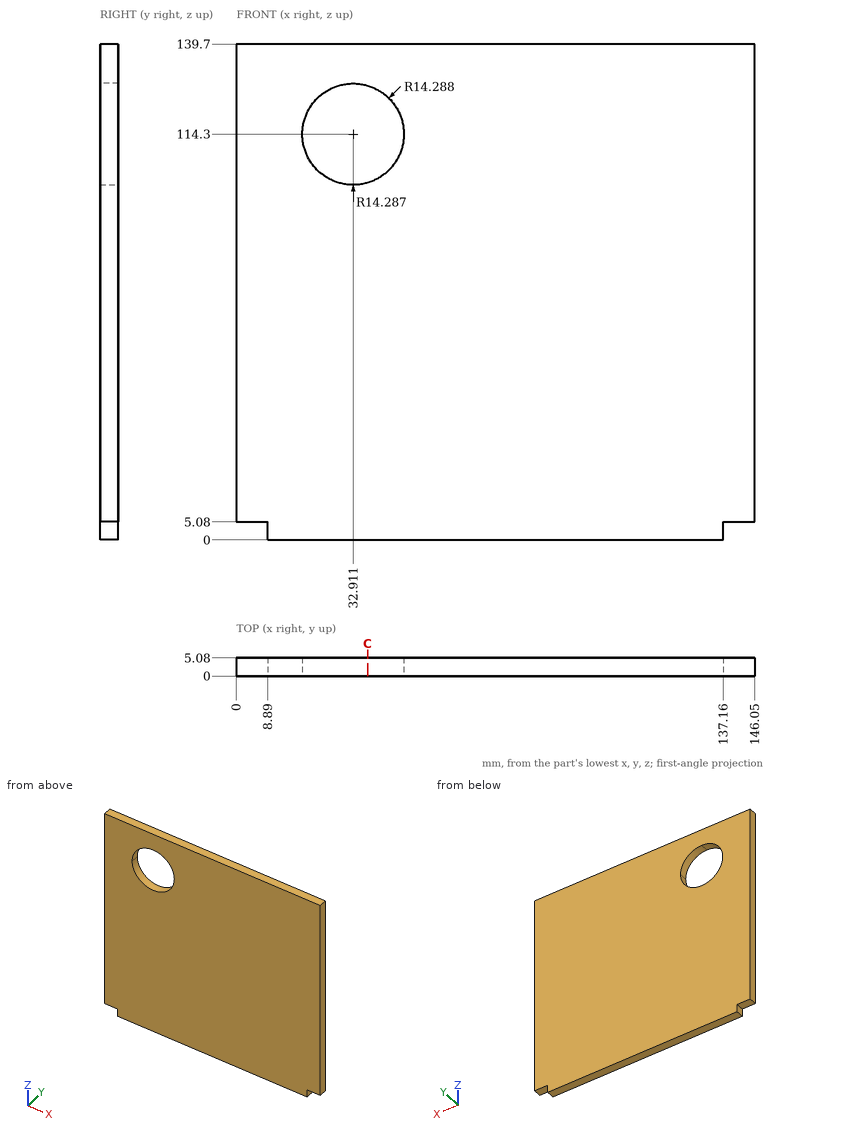
Answer from the drawing. Dimensions are ordinates in mm from the lowest x, y and z of the part. Round coordinates to 2 decimals unless told otherwise and drop trailing zeros. Loops run counter-clockwise (first coordinate to the right, second up) from the corner with the lowest first, then second, coordinate; pieces in that order, holes last.
Q1. Each of these flat-tipped pins is pushed along its axis until it touches: pin 1 (3 mm diameter, centred on x = 81, y = 1, fed in from -Z); pin 2 (1.5 mm diameter, centred on y = 2, z = 3.5, fed in from +X); pin 3 (1.5 mm diameter, centred on x = 3, y = 2, fed in from -Z). Where does it stop, or does it pass through?
Q2. Consider probe 1 along Z at (x, y) = (8, 4); probe 2 along Z at (x, y) = (42, 3.05) (1 decimal); probe 3 along Z at (x, y) = (37, 3.4). Determine where each line is inside the solid, lowest interval first.
Q3. Section C-C on x = 37 is taken. Write down the section's boundary in (y, z).
Output:
1. pin 1: stops at z = 0
1. pin 2: stops at x = 137.16
1. pin 3: stops at z = 5.08
2. probe 1: z = 5.08 to 139.7
2. probe 2: z = 0 to 103.3, 125.3 to 139.7
2. probe 3: z = 0 to 100.61, 127.99 to 139.7
3. outline: (0, 0) - (5.08, 0) - (5.08, 100.61) - (0, 100.61) - close; (0, 127.99) - (5.08, 127.99) - (5.08, 139.7) - (0, 139.7) - close
